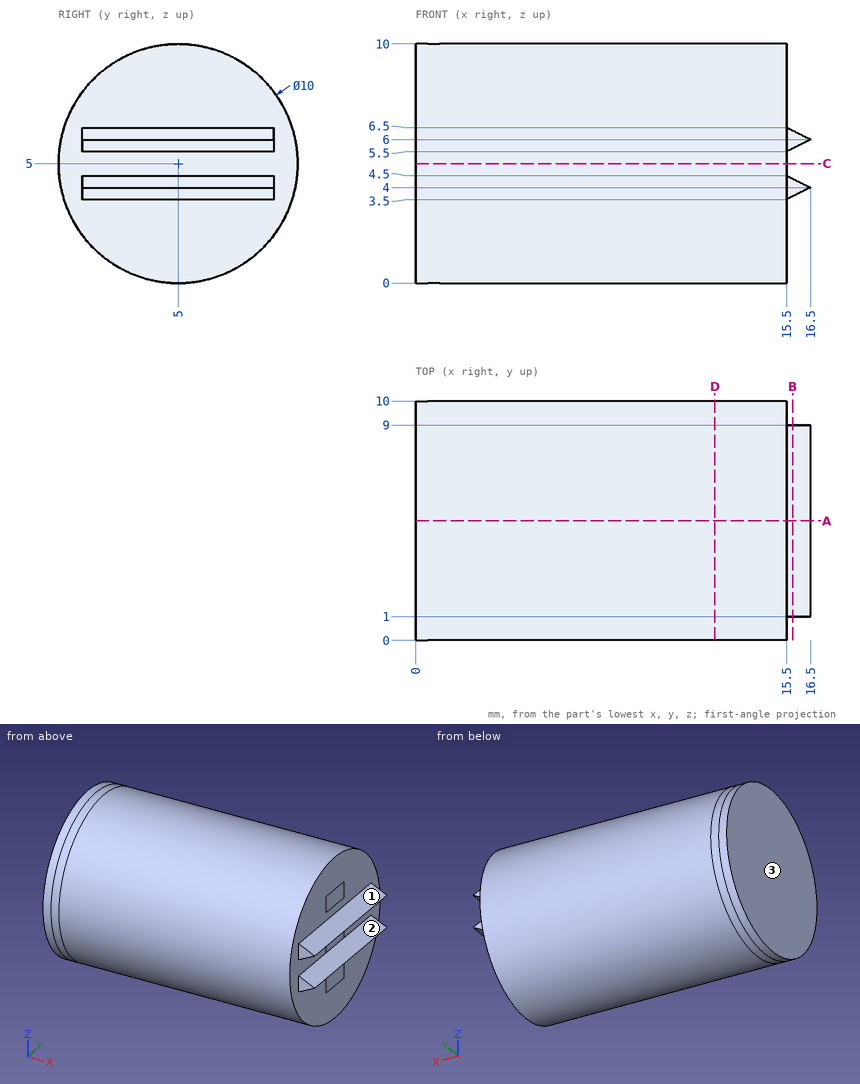
Could you check a few things on this drawing? It's one solid part, dimensions in mm from its lowest x, y, z. Give positions to 0.01 mm unless a question says otherwise; leave off trailing zeros. Order: outer loops, then holes, each group sorted by start corner. A loop starts at its lowest first (then second) coordinate and runs counter-clockwise, first axis right, second up. Notation, with made-up numbers: (-14, 6) - (21, 6) arc R20 ccw to (21, 38) - close; hole circle Ø5 at (-39, -39). An arc over 180 degrees is marked (long way). Return JSON: item names as keys, results as strings. Group by question number.
Q1. Suppose I cut it at A-A, the plane y = 5. Please give me the cut outline in (x, z), and give its area (3 significant figures).
Q2. Please list where these lines run through material, in increasing order: line 1 along X through (y, z) = (1.5, 3.25); line 2 along Y through (x, z) = (12.5, 1). Write a range as [from, to].
Q3. Will these pins go through, and if not, where does the flat tip stop? pin 1 Ø5 at (x, y) = (3, 8) entering from +Z; pin 2 Ø1.1 at (x, z) = (16, 4) entering from +Y; pin 3 Ø0.8 at (y, z) = (5, 2.5) entering from +X.
Q4. Suppose I cut it at C-C, the plane z = 5. Please give me the cut outline in (x, y).
Q5. Thinking about a two-plate mould opening in Z: for the marked faces 1, 2 and 3, which applies, pulls with the +Z half, pulls with the -Z half, needs draft (parallel to the pull), parting line crosses it, or undercut?
Q6. Suppose I cut it at D-D, the plane x = 12.5. Please give me the cut outline in (y, z).
Q7. Suppose I cut it at B-B, the plane x = 15.75. Please give me the cut outline in (y, z) (3 decimals).
Resolved:
{
 "1": {"outline": "(0, 0) - (15.5, 0) - (15.5, 3.5) - (16.5, 4) - (15.5, 4.5) - (15.5, 5.5) - (16.5, 6) - (15.5, 6.5) - (15.5, 10) - (0, 10) - close", "area": "156 mm2"},
 "2": {"line 1": "x = [0, 15.5]", "line 2": "y = [2, 8]"},
 "3": {"pin 1": "stops at z = 9.97", "pin 2": "stops at y = 9.94", "pin 3": "stops at x = 15.5"},
 "4": {"outline": "(0, 0) - (15.5, 0) - (15.5, 10) - (0, 10) - close"},
 "5": {"face 1": "pulls with the +Z half", "face 2": "undercut", "face 3": "needs draft"},
 "6": {"outline": "circle Ø10 at (5, 5)"},
 "7": {"outline": "(1, 3.625) - (9, 3.625) - (9, 4.375) - (1, 4.375) - close; (1, 5.625) - (9, 5.625) - (9, 6.375) - (1, 6.375) - close"}
}
